The listing builds one solid part. Answer for the finished solid, in the listing's coordinates (mm). A direction names the side the tool comes from. Give positions to 0.01 mm unless a question says otherwise; leave off trailing zeros. Write each loop counter-clockwise with the first axis right and the second up, starting at its lowest first coordinate (ties: lowest second). Pieces come first, ordered by that corner, then holes. Notation, with made-up numbers: (-35, 1.25) - (6, 1.25) arc R25 cw to (6, 34.25) - close; hole circle Ø10 at (-24, 38). An arc over 180 degrees is marked (long way). Answer in a Markdown table with one row per item. Add a question column.
Autodesk Inventor part; units mm, degrees
ref_plane "YZ Plane" through (0, 0, 0) normal (1, 0, 0) x (0, 1, 0)
ref_plane "XZ Plane" through (0, 0, 0) normal (0, 1, 0) x (-1, 0, 0)
ref_plane "XY Plane" through (0, 0, 0) normal (0, 0, 1) x (1, 0, 0)
sketch "Sketch1" plane through (0, 0, 0) normal (0, 0, 1) x (1, 0, 0)
  circle A0 centre (0, 0) radius 1.5875
  dimension "d0" = 3.175
extrude "Extrusion1" add sketch "Sketch1" along normal blind 3.81
sketch "Sketch2" plane through (0, 0, 3.81) normal (0, 0, 1) x (1, 0, 0)
  line L0 (2.54, 0) -> (1.27, -2.1997)
  line L1 (1.27, -2.1997) -> (-1.27, -2.1997)
  line L2 (-1.27, -2.1997) -> (-2.54, 0)
  line L3 (-2.54, 0) -> (-1.27, 2.1997)
  line L4 (-1.27, 2.1997) -> (1.27, 2.1997)
  line L5 (1.27, 2.1997) -> (2.54, 0)
  point P0 (0, 0)
  point P1 (0, 0)
  dimension "d5" = 5.08
extrude "Extrusion2" add sketch "Sketch2" along normal blind 1
thread "Thread1"
properties part number "Pedal Bar Bolt"
1. Section C-C (z = 2.1) is taken. Give the vertices of the cut face in (x, y) (1 decimal), and give its area (3 significant figures).
2. Section A-A (x = 0) is taken. Give the vertices of the cut face in (y, z), and give its area (3 significant figures).
3. Section D-D (y = -1.7) is taken. Give the vertices of the cut face in (x, z).
4. Section B-B (y = -0.4) is taken. Give the vertices of the cut face in (x, z), and give its area (3 significant figures).
5. A tool of negligible diameter and unlimited length cuts with its end or side. For faces 1 (the face through (2, 0, 3.81)), 2 (the face through (1.896, 1.115, 4.303)), from which of +Z, -Z, +X, -X, +Y, -Y can it reach the whole face along a straight path? Write none if from no direction.
6. Straight lines are drawn through the part: L1, parallel to Z at x = -0.4, y = -1.8; L2, parallel to Y at x = 0.2, z = 3.3; L3, parallel to Y at x = -1.05, z = 2.25. For each, find the intervals that lie inside material, in ascending order. Write a range as [from, to].
Geometry check:
| question | item | result |
|---|---|---|
| 1 | outline | circle Ø3.2 at (0, 0) |
| 1 | area | 7.92 mm² |
| 2 | outline | (-2.2, 3.81) - (-1.59, 3.81) - (-1.59, 0) - (1.59, 0) - (1.59, 3.81) - (2.2, 3.81) - (2.2, 4.81) - (-2.2, 4.81) - close |
| 2 | area | 16.5 mm² |
| 3 | outline | (-1.56, 3.81) - (1.56, 3.81) - (1.56, 4.81) - (-1.56, 4.81) - close |
| 4 | outline | (-2.31, 3.81) - (-1.54, 3.81) - (-1.54, 0) - (1.54, 0) - (1.54, 3.81) - (2.31, 3.81) - (2.31, 4.81) - (-2.31, 4.81) - close |
| 4 | area | 16.3 mm² |
| 5 | face 1 | -Z |
| 5 | face 2 | +Z, -Z, +X, +Y |
| 6 | L1 | [3.81, 4.81] |
| 6 | L2 | [-1.57, 1.57] |
| 6 | L3 | [-1.19, 1.19] |
